from build123d import *

# Parameters (mm, degrees)
SKETCH1_R           = 4.826
BOSS_EXTRUDE1_DEPTH = 30.988
SKETCH2_R           = 4.325
CUT_EXTRUDE1_DEPTH  = 37
SKETCH3_R           = 4.826
SKETCH3_R_2         = 4.325
CUT_EXTRUDE2_DEPTH  = 9.652
SKETCH5_R           = 4.325
SKETCH5_R_2         = 3.81
BOSS_EXTRUDE3_DEPTH = 0.635


with BuildPart() as part:
    # Sketch1 → Boss-Extrude1 (new body)
    with BuildSketch(Plane.XY):
        Circle(SKETCH1_R)
    extrude(amount=BOSS_EXTRUDE1_DEPTH)

    # Sketch2 → Cut-Extrude1 (cut)
    with BuildSketch(Plane.XY.offset(30.988)):
        Circle(SKETCH2_R)
    extrude(amount=-CUT_EXTRUDE1_DEPTH, mode=Mode.SUBTRACT)

    # Sketch3 → Cut-Extrude2 (cut)
    with BuildSketch(Plane.XY.offset(30.988)):
        Circle(SKETCH3_R)
        Circle(SKETCH3_R_2, mode=Mode.SUBTRACT)
    extrude(amount=-CUT_EXTRUDE2_DEPTH, mode=Mode.SUBTRACT)

    # Sketch5 → Boss-Extrude3 (add)
    with BuildSketch(Plane(origin=(0, 0, 7.874), x_dir=(-1, 0, 0), z_dir=(0, 0, -1))):
        Circle(SKETCH5_R)
        Circle(SKETCH5_R_2, mode=Mode.SUBTRACT)
    extrude(amount=-BOSS_EXTRUDE3_DEPTH)


solid = part.part
Design review of the part built by this model. Coordinates are the model's own, in mm. A direction names the side the tool comes from. Give positions to 0.01 mm unless a question says otherwise; leave off trailing zeros. Order: outer loops, then holes, each group sorted by start corner. A loop starts at its lowest first (then second) coordinate and runs counter-clockwise, first axis right, second up.
1. Tool access review of faces 3 (the cylindrical face through (4.125, 1.299, 15.012)), 4 (the cylindrical face through (4.125, 1.299, 3.992)), 5 (the cylindrical face through (0.83, -3.72, 8.19)): name each direction out of +Z, -Z, +X, -X, +Y, -Y from which nothing blocks a thin tool from reaching the whole face with its end or side.
Solution:
face 3: +Z
face 4: -Z
face 5: +Z, -Z
2. Add section C-C, the plane z = 2.5. State the section outline as (x, y) points (3 decimals).
Solution:
outline: circle Ø9.652 at (0, 0); hole circle Ø8.65 at (0, 0)
3. Mouldability with a two-part tool opening along Y and no side actions: class faces 1 (the flat face through (0, -4, 7.874)), 2 (the cylindrical face through (-3.83, -2.937, 10.519)) as +Y half, -Y half, draft (parallel to the pull), parting line (faces both ways), or undercut.
Solution:
face 1: undercut
face 2: parting line
4. Add section A-A, the plane x = 0. State the section outline as (y, z) points (3 decimals).
Solution:
outline: (-4.826, 0) - (-4.325, 0) - (-4.325, 7.874) - (-3.81, 7.874) - (-3.81, 8.509) - (-4.325, 8.509) - (-4.325, 21.336) - (-4.826, 21.336) - close; (3.81, 7.874) - (4.325, 7.874) - (4.325, 0) - (4.826, 0) - (4.826, 21.336) - (4.325, 21.336) - (4.325, 8.509) - (3.81, 8.509) - close
5. To check wall thickness, follow L1, parallel to Y at x = 0, z = 11.5 (3 decimals); L2, parallel to Y at x = 0, z = 8.3; L3, parallel to X at y = -2, z = 9.75. State the ranges of each line that lie inside material, in increasing order.
Solution:
L1: y = -4.826 to -4.325, 4.325 to 4.826
L2: y = -4.83 to -3.81, 3.81 to 4.83
L3: x = -4.39 to -3.83, 3.83 to 4.39
6. For pin 1 Ø4.5 at (x, y) = (0.5, 0) entering from -Z (3 decimals); pin 2 Ø2 at (y, z) = (3.5, 16) entering from -X, all flat-tipped, find the tip position at first contact; note any pin that passes through.
Solution:
pin 1: passes through
pin 2: stops at x = -4.13
